Work out the finished part from the listing and answer in its coordinate system (mm). A direction names the side the tool comes from. Give positions to 0.01 mm unless a question says otherwise; leave off trailing zeros. Order: outer loops, then holes, each group sorted by start corner. A loop starts at its lowest first (then second) coordinate and runs counter-clockwise, first axis right, second up.
```python
from build123d import *

# Parameters (mm, degrees)
BOSS_EXTRUDE1_DEPTH = 40
CUT_EXTRUDE1_DEPTH  = 35
CHAMFER1_SIZE       = 20
SKETCH4_R           = 5
CUT_EXTRUDE2_DEPTH  = 77.485292704
FILLET1_R           = 2
CHAMFER2_SIZE       = 0.5


with BuildPart() as part:
    # Sketch1 → Boss-Extrude1 (new body)
    with BuildSketch(Plane(origin=(0, 0, 0), x_dir=(1, 0, 0), z_dir=(0, 1, 0))):
        Polygon((-35, -30), (-35, 30), (-15, 25), (15, 25), (35, 30), (35, -30), (15, -25), (-15, -25), align=None)
    extrude(amount=BOSS_EXTRUDE1_DEPTH)

    # Sketch2 → Cut-Extrude1 (cut)
    with BuildSketch(Plane(origin=(0, 40, 0), x_dir=(1, 0, 0), z_dir=(0, 1, 0))):
        Polygon((-15.369316877, 22), (-49.922572363, 30.638313872), (-49.922572363, -30.638313872), (-15.369316877, -22), (15.369316877, -22), (46.296501907, -29.731796258), (46.296501907, 29.731796258), (15.369316877, 22), align=None)
    extrude(amount=-CUT_EXTRUDE1_DEPTH, mode=Mode.SUBTRACT)

    # Chamfer1
    # the kernel refuses this chamfer: 20 mm, written as the material it takes off along each edge
    with BuildSketch(Plane(origin=(35, 40, -24.525988979), x_dir=(-0.9996219169112968, 0.027495876610586317, 0), z_dir=(0, 0, 1)), Plane(origin=(35, 40, -81.433659759), x_dir=(-0.9996219169112968, 0.027495876610586317, 0), z_dir=(0, 0, 1))) as chamfer1_piece_1:
        Polygon((CHAMFER1_SIZE * 0.999621916911, CHAMFER1_SIZE * 0.0274958766106), (-CHAMFER1_SIZE * 0.0274958766106, CHAMFER1_SIZE * 0.999621916911), (0, 0), align=None)
    extrude(amount=105.959648738, mode=Mode.SUBTRACT)
    with BuildSketch(Plane(origin=(-35, 40, 24.525988979), x_dir=(-0.027495876610586317, -0.9996219169112968, 0), z_dir=(0, 0, -1)), Plane(origin=(-35, 40, 81.433659759), x_dir=(-0.027495876610586317, -0.9996219169112968, 0), z_dir=(0, 0, -1))) as chamfer1_piece_2:
        Polygon((CHAMFER1_SIZE * 0.999621916911, -CHAMFER1_SIZE * 0.0274958766106), (-CHAMFER1_SIZE * 0.0274958766106, -CHAMFER1_SIZE * 0.999621916911), (0, 0), align=None)
    extrude(amount=105.959648738, mode=Mode.SUBTRACT)

    # Sketch4 → Cut-Extrude2 (cut, through all)
    with BuildSketch(Plane.XY.offset(25)):
        with Locations((0, 25)):
            Circle(SKETCH4_R)
    extrude(amount=-CUT_EXTRUDE2_DEPTH, mode=Mode.SUBTRACT)

    # Fillet1
    fillet1_edges = [part.edges().sort_by_distance(p)[0] for p in [
        (25.184658438, 5, -24.45383539),
        (25.184658438, 5, 24.45383539),
        (-25.184658438, 5, 24.45383539),
        (-25.184658438, 5, -24.45383539),
        (0, 5, -22),
        (0, 5, 22),
    ]]
    fillet(fillet1_edges, radius=FILLET1_R)

    # Chamfer2
    chamfer2_edges = [part.edges().sort_by_distance(p)[0] for p in [
        (-5, 25, -22),
        (-5, 25, -25),
        (-5, 25, 22),
        (-5, 25, 25),
    ]]
    chamfer(chamfer2_edges, length=CHAMFER2_SIZE)


solid = part.part
```
1. The part is cut by section B-B (y = 9.5). Write down the section's boundary in (x, z).
Findings below:
outline: (-35, -30) - (-15, -25) - (15, -25) - (35, -30) - (35, -26.91) - (15.37, -22) - (-15.37, -22) - (-35, -26.91) - close; (-35, 26.91) - (-15.37, 22) - (15.37, 22) - (35, 26.91) - (35, 30) - (15, 25) - (-15, 25) - (-35, 30) - close
2. The mould has two halves that part along Z. Classify faces 1 (the face through (-24.86, 15.276, 27.465)), 2 (the face through (-22.866, 19.918, -23.874)), 3 (the face through (-1.08, 20.12, -23.49)), 4 (the face through (-25.072, 5.57, 23.806)): pulls with the +Z half, pulls with the -Z half, needs draft (parallel to the pull), parting line crosses it, or undercut.
Findings below:
face 1: pulls with the +Z half
face 2: undercut
face 3: needs draft
face 4: undercut
3. Given P1, Ø2, axis at x = -23, z = -22, coming from the +Y side; P2, Ø2, axis at x = -24.5, z = 1, coming from the +Y side; P3, Ø9, axis at x = -5, y = 19.5, coming from the +Z side, each flat-ended and moving along its own axis, determine where each tip first touches the part or whether it passes through.
Findings below:
P1: stops at y = 5.36
P2: stops at y = 5
P3: stops at z = 25
4. Straight lines are drawn through the part: probe 1 along Y at (x, z) = (0, 23); probe 2 along Y at (x, z) = (-9.5, 14); probe 3 along Z at (x, y) = (0.5, 30.5). For each, find the intervals that lie inside material, in ascending order.
Findings below:
probe 1: y = 0 to 20, 30 to 40
probe 2: y = 0 to 5
probe 3: z = -25 to -22, 22 to 25
5. The part is cut by section C-C (x = -10.5). Write down the section's boundary in (y, z).
Findings below:
outline: (0, -25) - (40, -25) - (40, -22) - (7, -22) arc R2 cw to (5, -20) - (5, 20) arc R2 cw to (7, 22) - (40, 22) - (40, 25) - (0, 25) - close
6. Which of the six approach directions +Z, -Z, +X, -X, +Y, -Y give full straight-line access (tool end or side, diameter ignored) to faces 5 (the face through (-23.141, 19.918, 23.943)), 6 (the face through (4, 20, 25)), 7 (the face through (25.35, 5.57, 23.875))?
Findings below:
face 5: -X, +Y
face 6: +Z, +Y, -Y
face 7: +X, +Y
7. The part is cut by section D-D (y = 25). State how many separate pieces and enclosed holes the cut face has, then the cut area to 3 significant figures.
Findings below:
separate pieces: 4
enclosed holes: 0
area: 304 mm2
8. The part is cut by section A-A (x = 0). Write down the section's boundary in (y, z), then the cut area to 3 significant figures.
Findings below:
outline: (0, -25) - (19.5, -25) - (20, -24.5) - (20, -22.5) - (19.5, -22) - (7, -22) arc R2 cw to (5, -20) - (5, 20) arc R2 cw to (7, 22) - (19.5, 22) - (20, 22.5) - (20, 24.5) - (19.5, 25) - (0, 25) - close; (30, -24.5) - (30.5, -25) - (40, -25) - (40, -22) - (30.5, -22) - (30, -22.5) - close; (30, 22.5) - (30.5, 22) - (40, 22) - (40, 25) - (30.5, 25) - (30, 24.5) - close
area: 401 mm2
